For this review, take the finished solid that the model builds, in its own axes (mm). Coordinates: 2 decimals unless noted, no trailing zeros. Loops run counter-clockwise (first coordinate to the right, second up) from the corner with the lowest first, then second, coordinate; pieces in that order, holes last. Notation, with made-up numbers: M 81.5,65.25 L 118.5,65.25 A9 ccw 118.5,74.25 Z; hole C 56.5,82 d2. An arc over 180 degrees is marked long. Answer as a JSON object with one key per item and string values. Group by question number.
Item 1: Wall thickness on L1, parallel to X at y = 18.5, z = -13; L2, parallel to Z at x = 0.5, y = 11; L3, parallel to Z at x = -4, y = 11: over which ranges is each line inside the solid? List them lowest first. Write a range as from..to.
Item 2: Add section C-C (x = 12). State the section outline as (y, z) points.
Item 3: Mouldability with a two-part tool opening along Z and no side actions: class faces 1 (the face through (8.438, 14.282, -15.956)), 2 (the face through (-8.937, 14.17, -15.074)) as +Z half, -Z half, draft (parallel to the pull), parting line (faces both ways), or undercut.
Item 4: Insertion check: pin 1 (8 mm diameter, centred on x = -18.5, y = 2, fed in from -Z); pin 2 (12 mm diameter, centred on x = 3.5, y = -17, fed in from +Z); pin 3 (13 mm diameter, centred on x = 3, y = 15, fed in from -Z). Each pin has a flat end and moves straight along its axis. Give the tip position at first contact, or say it passes through.
Item 5: Add section D-D (y = 3.5). State the section outline as (x, z) points, then the cut area to 3 significant figures.
Item 6: Add section A-A (y = 15.5). State the section outline as (x, z) points, then the cut area to 3 significant figures.
Item 7: Add section B-B (z = -20). State the section outline as (x, y) points.
from build123d import *

# Parameters (mm, degrees)
SKETCH_6_W          = 13.38221488
SKETCH_6_H          = 4.41838063
CUT_EXTRUDE_1_DEPTH = 50.749371855


with BuildPart() as part:
    # 草图4 → 旋转1 (revolve)
    with BuildSketch(Plane(origin=(0, 0, 0), x_dir=(0, 0, -1), z_dir=(1, 0, 0))):
        with BuildLine():
            Line((0, -25), (0, 0))
            Line((0, 0), (0, 17.552013601))
            Line((0, 17.552013601), (0, 25))
            ThreePointArc((0, 25), (-25, 0), (0, -25))
        make_face()
    revolve(axis=Axis((0, 0, 0), (0, 1, 0)))

    # 草图6 → 切除-拉伸1 (cut, through all)
    with BuildSketch(Plane(origin=(0, 10, 0), x_dir=(1, 0, 0), z_dir=(0, 1, 0))):
        with BuildLine():
            Line((-14.30889256, 11.940688041), (-13.30889256, 11.940688041))
            ThreePointArc((-13.30889256, 11.940688041), (-10, 15.2495806), (-6.69110744, 11.940688041))
            Line((-6.69110744, 11.940688041), (-5.69110744, 11.940688041))
            ThreePointArc((-5.69110744, 11.940688041), (-10, 16.2495806), (-14.30889256, 11.940688041))
        make_face()
        with Locations((0, -10.364363226)):
            Rectangle(SKETCH_6_W, SKETCH_6_H)
        with BuildLine():
            ThreePointArc((5.69110744, 11.940688041), (10, 16.2495806), (14.30889256, 11.940688041))
            Line((14.30889256, 11.940688041), (13.30889256, 11.940688041))
            ThreePointArc((13.30889256, 11.940688041), (10, 15.2495806), (6.69110744, 11.940688041))
            Line((6.69110744, 11.940688041), (5.69110744, 11.940688041))
        make_face()
    extrude(amount=CUT_EXTRUDE_1_DEPTH, mode=Mode.SUBTRACT)


solid = part.part
From the geometry:
{
 "1": {"L1": "x = -10.67..-6.87, -5.82..5.82, 6.87..10.67", "L2": "z = -22.44..8.16, 12.57..22.44", "L3": "z = -22.09..8.16, 12.57..22.09"},
 "2": {"outline": "M 10,-15.76 L 10,-14.58 L 16.39,-14.58 A21.93 ccw long 15.25,-15.76 Z"},
 "3": {"face 1": "undercut", "face 2": "undercut"},
 "4": {"pin 1": "stops at z = -20.29", "pin 2": "stops at z = 22.27", "pin 3": "stops at z = -23.4"},
 "5": {"outline": "C 0,0 d49.51", "area": "1,930 mm²"},
 "6": {"outline": "M -14.31,-11.94 L -13.31,-11.94 A3.31 ccw -6.69,-11.94 L -5.69,-11.94 A4.31 cw -11.26,-16.06 A19.62 ccw 11.26,-16.06 A4.31 cw 5.69,-11.94 L 6.69,-11.94 A3.31 ccw 13.31,-11.94 L 14.31,-11.94 A4.31 cw 13.84,-13.9 A19.62 ccw long -13.84,-13.9 A4.31 cw Z; hole M -6.69,8.16 L 6.69,8.16 L 6.69,12.57 L -6.69,12.57 Z", "area": "1,130 mm²"},
 "7": {"outline": "C 0,0 d30"}
}
